Input: part model. Units: mm. Frame: model coordinates. Face numbers are marked on the shaded views. Round coordinates to 2 decimals unless told otherwise and drop trailing zeros. Write each loop counter-clockwise with the first axis right and the second up, starting at its lowest first coordinate (ties: lowest second). Pieces come first, ordered by that corner, then holes. Notation, with made-up numbers: (-3, 79.25) -> (42, 79.25) arc R19 ccw to (42, 99.25) -> close; hole circle Ø2 at (-17.75, -25). An arc over 180 degrees is marked (long way). Write item = value, one per line.
```python
from build123d import *
from OCP.BRepFilletAPI import BRepFilletAPI_MakeChamfer

# Parameters (mm, degrees)
ESQUISSE1_W        = 70
ESQUISSE1_H        = 70
BOSS_EXTRU_1_DEPTH = 4
BOSS_EXTRU_2_DEPTH = 4.6
BOSS_EXTRU_3_DEPTH = 3
CHANFREIN1_SIZE    = 2
CHANFREIN1_SIZE2   = 6
CHANFREIN2_SIZE    = 25


with BuildPart() as part:
    # Esquisse1 → Boss.-Extru.1 (new body)
    with BuildSketch(Plane.XY):
        Rectangle(ESQUISSE1_W, ESQUISSE1_H)
    extrude(amount=BOSS_EXTRU_1_DEPTH)

    # Esquisse2 → Boss.-Extru.2 (add)
    with BuildSketch(Plane.XY.offset(4)):
        Polygon((-35, 35), (-35, -35), (-32, -35), (-32, 32), (35, 32), (35, 35), align=None)
    extrude(amount=BOSS_EXTRU_2_DEPTH)

    # Esquisse3 → Boss.-Extru.3 (add)
    with BuildSketch(Plane.XY.offset(8.6)):
        with BuildLine():
            Line((35, 35), (-35, 35))
            Line((-35, 35), (-35, -35))
            Line((-35, -35), (-27, -35))
            Line((-27, -35), (-27, -30))
            ThreePointArc((-27, -30), (-20.095113441, -27.13990234), (-17.235015781, -20.235015781))
            Line((-17.235015781, -20.235015781), (-12.235015781, -20.235015781))
            ThreePointArc((-12.235015781, -20.235015781), (-2.207811813, 3.972796032), (22, 14))
            Line((22, 14), (22, 19))
            ThreePointArc((22, 19), (27.656854249, 21.343145751), (30, 27))
            Line((30, 27), (35, 27))
            Line((35, 27), (35, 35))
        make_face()
    extrude(amount=BOSS_EXTRU_3_DEPTH)

    # Chanfrein1: one chamfer whose edges measure the first distance from different faces: ONE call of the kernel's chamfer builder (chamfer() names one face for all edges)
    chanfrein1_edges_1 = [part.edges().sort_by_distance(p)[0] for p in [
        (0, 35, 11.6),
    ]]
    chanfrein1_side_1 = [part.faces().sort_by_distance(p)[0] for p in [
        (0, 35, 5.8),
    ]]
    chanfrein1_edges_2 = [part.edges().sort_by_distance(p)[0] for p in [
        (-35, 0, 11.6),
    ]]
    chanfrein1_side_2 = [part.faces().sort_by_distance(p)[0] for p in [
        (-35, 0, 5.8),
    ]]
    chanfrein1 = BRepFilletAPI_MakeChamfer(part.part.solid().wrapped)
    for e in chanfrein1_edges_1:
        chanfrein1.Add(CHANFREIN1_SIZE, CHANFREIN1_SIZE2, e.wrapped, chanfrein1_side_1[0].wrapped)  # the first distance lies on this face
    for e in chanfrein1_edges_2:
        chanfrein1.Add(CHANFREIN1_SIZE, CHANFREIN1_SIZE2, e.wrapped, chanfrein1_side_2[0].wrapped)  # the first distance lies on this face
    add(Compound.cast(chanfrein1.Shape()), mode=Mode.REPLACE)

    # Chanfrein2
    chanfrein2_edges = [part.edges().sort_by_distance(p)[0] for p in [
        (35, -35, 2),
    ]]
    chamfer(chanfrein2_edges, length=CHANFREIN2_SIZE)

    # Esquisse4 → Fraisage pour vis à tête fraisée M51 (revolve, cut)
    with BuildSketch(Plane(origin=(10, -10, 4), x_dir=(0, -1, 0), z_dir=(1, 0, 0))):
        Polygon((0, 0), (0, 4), (2.75, 4), (2.75, 2.45), (5.2, 0), align=None)
    revolve(axis=Axis((10, -10, 10.35), (0, 0, -1)), mode=Mode.SUBTRACT)


solid = part.part
```
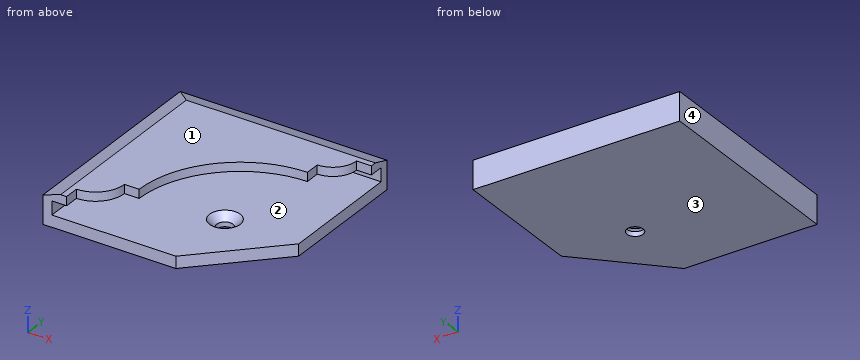
1) Cut plane D-D (z = 10.5). Return the cut outline in (x, y).
Solutions:
outline = (-32.3, -35) -> (-27, -35) -> (-27, -30) arc R9.76 ccw to (-17.24, -20.24) -> (-12.24, -20.24) arc R34.24 cw to (22, 14) -> (22, 19) arc R8 ccw to (30, 27) -> (35, 27) -> (35, 32.3) -> (-32.3, 32.3) -> close
2) Cut plane A-A (y = 30.5). Return the cut outline in (x, z), and give its area (3 significant figures).
Solutions:
outline = (-35, 0) -> (35, 0) -> (35, 4) -> (-32, 4) -> (-32, 8.6) -> (35, 8.6) -> (35, 11.1) -> (-30.5, 11.1) -> (-35, 9.6) -> close
area = 465 mm^2
3) Line query: L1, parallel to Z at x = -10, y = 10.5; L2, parallel to Y at x = 10, z = 1.15; L3, parallel to Z at x = 30.5, y = 16.5. Output: solid intervals per line, ascending. Write a range as from..to.
Solutions:
L1 = 0..4, 8.6..11.6
L2 = -35..-12.75, -7.25..35
L3 = 0..4
4) Draft query along Z for the marked faces 1, 2, 3 and 4. Return one class per face: +Z half, -Z half, draft (parallel to the pull), parting line (faces both ways), or undercut.
Solutions:
face_1 = +Z half
face_2 = undercut
face_3 = -Z half
face_4 = draft
5) Cut plane C-C (x = -24). Return the cut outline in (y, z).
Solutions:
outline = (-35, 0) -> (35, 0) -> (35, 9.6) -> (29, 11.6) -> (-29.53, 11.6) -> (-29.53, 8.6) -> (32, 8.6) -> (32, 4) -> (-35, 4) -> close
6) First-contact query: P1, Ø0.9, axis at x = 31.5, z = 9.5, coming from the -Y side; P2, Ø6, axis at x = -6.5, y = -18.5, coming from the +Z side; P3, Ø1.4, axis at x = 0.5, z = 6.5, coming from the -Y side. Flat tips, straight axial feed; report the tip coordinate or a pass-through.
Solutions:
P1 = 27
P2 = 4
P3 = 32
7) Cut plane B-B (z = 2.5). Return the cut outline in (x, y).
Solutions:
outline = (-35, -35) -> (10, -35) -> (35, -10) -> (35, 35) -> (-35, 35) -> close; hole circle Ø7.4 at (10, -10)
